from build123d import *

# Parameters (mm, degrees)
SKETCH1_W           = 60
SKETCH1_H           = 4
BOSS_EXTRUDE1_DEPTH = 25
SKETCH2_W           = 50
SKETCH2_H           = 5.5
BOSS_EXTRUDE2_DEPTH = 60
FILLET1_R           = 5
SKETCH3_R           = 4
CUT_EXTRUDE1_DEPTH  = 60


with BuildPart() as part:
    # Sketch1 → Boss-Extrude1 (new body)
    with BuildSketch(Plane.XY):
        with Locations((0, 0.807157058)):
            Rectangle(SKETCH1_W, SKETCH1_H)
    extrude(amount=BOSS_EXTRUDE1_DEPTH)

    # Sketch2 → Boss-Extrude2 (add)
    with BuildSketch(Plane(origin=(0, 2.807157058, 0), x_dir=(1, 0, 0), z_dir=(0, 1, 0))):
        with Locations((0, -12.5)):
            Rectangle(SKETCH2_W, SKETCH2_H)
    extrude(amount=BOSS_EXTRUDE2_DEPTH)

    # Fillet1
    fillet1_edges = [part.edges().sort_by_distance(p)[0] for p in [
        (25, 2.807157058, 12.5),
        (0, 2.807157058, 9.75),
        (-25, 2.807157058, 12.5),
        (0, 2.807157058, 15.25),
    ]]
    fillet(fillet1_edges, radius=FILLET1_R - 0.0001)  # a hair under: the kernel refuses the full size

    # Sketch3 → Cut-Extrude1 (cut)
    with BuildSketch(Plane.XY.offset(15.25)):
        with Locations((-11.715, 43.307157058)):
            Circle(SKETCH3_R)
        with Locations((11.715, 43.307157058)):
            Circle(SKETCH3_R)
    extrude(amount=-CUT_EXTRUDE1_DEPTH, mode=Mode.SUBTRACT)


solid = part.part
Source: CAD feature listing. Evaluate the final solid. Frame: model axes, mm. A direction names the side the tool comes from. Give positions to 0.01 mm unless a question says otherwise; leave off trailing zeros. Loops run counter-clockwise (first coordinate to the right, second up) from the corner with the lowest first, then second, coordinate; pieces in that order, holes last. Notation, with made-up numbers: (-9, 38) -> (35, 38) arc R29 cw to (35, 60) -> close; hole circle Ø1 at (-21, 5). An arc over 180 degrees is marked (long way). Use a Markdown table: item, result. Add a question column.
1) Section query A-A, the plane x = -12.5. Return the cut outline in (y, z), then the cut area to 3 significant figures.
2) Pull-direction query (X, two-part tool) for faces 1 (the face through (11.194, 47.273, 12.538)), 2 (the face through (27.18, 3.68, 12.39)), 3 (the face through (0, -1.193, 12)), 4 (the face through (-12.236, 47.273, 12.538)); classes: +X half, -X half, draft (parallel to the pull), parting line (faces both ways), or undercut.
3) Section query C-C, the plane z = 10.5. Count the separate pieces of the cut face and the enclosed holes in it, then the cut area to 3 significant figures.
4) Line query: line 1 along X through (y, z) = (40, 10); line 2 along Z through (x, y) = (22, 47); line 3 along Y through (x, z) = (10.5, 2.75). Output: solid intervals per line, ascending. Write a range as [from, to].
5) Reachability of faces 5 (the face through (25, 35, 13)), 6 (the face through (0, 35, 15.25)), 7 (the face through (0, 2.807, 21)) from +Z, -Z, +X, -X, +Y, -Y: full face, straight path, thin tool, end or side. Return the list, or none.
6) Section query B-B, the plane x = -5. Return the cut outline in (y, z), then the cut area to 3 significant figures.
7) First-contact query: pin 1 (4.5 mm diameter, centred on y = 43, z = 13.5, fed in from +X); pin 2 (12 mm diameter, centred on x = 13.5, y = 48, fed in from +Z); pin 3 (10 mm diameter, centred on x = -16, z = 5.5, fed in from +Y); pin 4 (1.6 mm diameter, centred on y = 34, z = 13, fed in from -X). Flat tips, straight axial feed; report the tip coordinate or a pass-through.
8) Section query D-D, the plane z = 21.5. Return the cut outline in (x, y).
Numbers:
| question | item | result |
|---|---|---|
| 1 | outline | (-1.19, 0) -> (2.81, 0) -> (2.81, 4.75) arc R5 cw to (7.81, 9.75) -> (39.38, 9.75) -> (39.38, 15.25) -> (7.81, 15.25) arc R5 cw to (2.81, 20.25) -> (2.81, 25) -> (-1.19, 25) -> close; (47.23, 9.75) -> (62.81, 9.75) -> (62.81, 15.25) -> (47.23, 15.25) -> close |
| 1 | area | 398 mm2 |
| 2 | face 1 | undercut |
| 2 | face 2 | +X half |
| 2 | face 3 | draft |
| 2 | face 4 | undercut |
| 3 | separate pieces | 1 |
| 3 | enclosed holes | 2 |
| 3 | area | 3,150 mm2 |
| 4 | line 1 | x = [-25, -13.97], [-9.46, 9.46], [13.97, 25] |
| 4 | line 2 | z = [9.75, 15.25] |
| 4 | line 3 | y = [-1.19, 2.81] |
| 5 | face 5 | +Z, -Z, +X, +Y |
| 5 | face 6 | +Z, +X, -X, +Y |
| 5 | face 7 | +X, -X, +Y |
| 6 | outline | (-1.19, 0) -> (2.81, 0) -> (2.81, 4.75) arc R5 cw to (7.81, 9.75) -> (62.81, 9.75) -> (62.81, 15.25) -> (7.81, 15.25) arc R5 cw to (2.81, 20.25) -> (2.81, 25) -> (-1.19, 25) -> close |
| 6 | area | 441 mm2 |
| 7 | pin 1 | stops at x = 25 |
| 7 | pin 2 | stops at z = 15.25 |
| 7 | pin 3 | stops at y = 62.81 |
| 7 | pin 4 | stops at x = -25 |
| 8 | outline | (-30, -1.19) -> (30, -1.19) -> (30, 2.81) -> (-30, 2.81) -> close |
